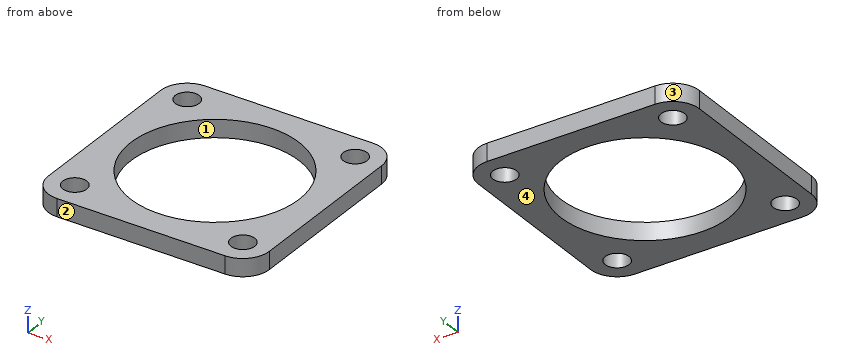
from build123d import *

# Parameters (mm, degrees)
SKETCH1_W           = 25
SKETCH1_H           = 25
SKETCH1_R           = 1.35
SKETCH1_R_2         = 9.5
BOSS_EXTRUDE1_DEPTH = 1
FILLET1_R           = 3


with BuildPart() as part:
    # Sketch1 → Boss-Extrude1 (new, symmetric)
    with BuildSketch(Plane.XY):
        Rectangle(SKETCH1_W, SKETCH1_H)
        with Locations((-9.5, 9.5)):
            Circle(SKETCH1_R, mode=Mode.SUBTRACT)
        with Locations((9.5, 9.5)):
            Circle(SKETCH1_R, mode=Mode.SUBTRACT)
        with Locations((9.5, -9.5)):
            Circle(SKETCH1_R, mode=Mode.SUBTRACT)
        with Locations((-9.5, -9.5)):
            Circle(SKETCH1_R, mode=Mode.SUBTRACT)
        Circle(SKETCH1_R_2, mode=Mode.SUBTRACT)
    extrude(amount=BOSS_EXTRUDE1_DEPTH, both=True)

    # Fillet1
    fillet1_edges = [part.edges().sort_by_distance(p)[0] for p in [
        (12.5, -12.5, 0),
        (-12.5, -12.5, 0),
        (-12.5, 12.5, 0),
        (12.5, 12.5, 0),
    ]]
    fillet(fillet1_edges, radius=FILLET1_R)


solid = part.part
Model file for the job. Use its own axes, mm. Face numbers are marked on the shaded views. Coordinates: 2 decimals unless noted, no trailing zeros. Order: outer loops, then holes, each group sorted by start corner. A loop starts at its lowest first (then second) coordinate and runs counter-clockwise, first axis right, second up. Notation, with made-up numbers: (-21.5, 55.25) -> (5.5, 55.25) arc R19 cw to (5.5, 67.25) -> close; hole circle Ø10 at (-19.5, -38.5). An arc over 180 degrees is marked (long way). Return JSON: item names as keys, results as strings. Group by question number.
Item 1: Saw through at A-A on x = 0. Write the cut outline in (y, z).
Item 2: Saw through at D-D on y = 11.25. Write the cut outline in (x, z).
Item 3: Pull direction Y, two halves, no side cores. Call the marked faces 1, 2, 3 and 4: pulls with the +Y half, pulls with the -Y half, needs draft (parallel to the pull), parting line crosses it, or undercut.
Item 4: Wall check: line 1 along Y through (x, z) = (0, 0.4); line 2 along X through (y, z) = (-6.75, 0.85); line 3 along X through (y, z) = (-2.5, 0.15). Give the ranges that are in metal, low to high. Write a range as [from, to].
Item 5: Flat gauge pin, fed straight in: P1, Ø2.5, axis at x = -9.5, y = -9.5, coming from the -Z side. Where does the tip first touch, or does it go through?
Item 6: Saw through at C-C on z = -0.5. Write the cut outline in (x, y), then the cut area to 3 significant figures.
Values found:
{
 "1": {"outline": "(-12.5, -1) -> (-9.5, -1) -> (-9.5, 1) -> (-12.5, 1) -> close; (9.5, -1) -> (12.5, -1) -> (12.5, 1) -> (9.5, 1) -> close"},
 "2": {"outline": "(-11.94, -1) -> (11.94, -1) -> (11.94, 1) -> (-11.94, 1) -> close"},
 "3": {"face 1": "undercut", "face 2": "pulls with the -Y half", "face 3": "pulls with the +Y half", "face 4": "needs draft"},
 "4": {"line 1": "y = [-12.5, -9.5], [9.5, 12.5]", "line 2": "x = [-12.5, -6.68], [6.68, 12.5]", "line 3": "x = [-12.5, -9.17], [9.17, 12.5]"},
 "5": {"P1": "passes through"},
 "6": {"outline": "(-12.5, -9.5) arc R3 ccw to (-9.5, -12.5) -> (9.5, -12.5) arc R3 ccw to (12.5, -9.5) -> (12.5, 9.5) arc R3 ccw to (9.5, 12.5) -> (-9.5, 12.5) arc R3 ccw to (-12.5, 9.5) -> close; hole circle Ø2.7 at (-9.5, -9.5); hole circle Ø2.7 at (-9.5, 9.5); hole circle Ø19 at (0, 0); hole circle Ø2.7 at (9.5, -9.5); hole circle Ø2.7 at (9.5, 9.5)", "area": "311 mm2"}
}
